```python
from build123d import *

# Parameters (mm, degrees)
F0_R     = 14
F1_DEPTH = 40
F2_R     = 2.5
F3_DEPTH = 15
F4_R     = 2.5
F5_DEPTH = 15


with BuildPart() as f1:
    # F0 (on Front) → F1 (new body)
    with BuildSketch(Plane.XZ):
        Polygon((0, 28), (0, 0), (52, 0), (52, 28), (40, 40), (12, 40), align=None)
        with Locations((26, 20)):
            Circle(F0_R, mode=Mode.SUBTRACT)
    extrude(amount=F1_DEPTH)

    # F2 (on face) → F3 (cut)
    with BuildSketch(Plane.XZ.offset(40)):
        with Locations((39.435029, 33.435029)):
            Circle(F2_R)
        with Locations((45, 20)):
            Circle(F2_R)
        with Locations((39.435029, 6.564971)):
            Circle(F2_R)
        with Locations((12.564971, 6.564971)):
            Circle(F2_R)
        with Locations((7, 20)):
            Circle(F2_R)
        with Locations((12.564971, 33.435029)):
            Circle(F2_R)
    extrude(amount=-F3_DEPTH, mode=Mode.SUBTRACT)

    # F4 (on face) → F5 (cut)
    with BuildSketch(Plane(origin=(0, 0, 0), x_dir=(1, 0, 0), z_dir=(0, 0, -1))):
        with Locations((46, 32)):
            Circle(F4_R)
        with Locations((46, 8)):
            Circle(F4_R)
        with Locations((6, 8)):
            Circle(F4_R)
        with Locations((6, 32)):
            Circle(F4_R)
    extrude(amount=-F5_DEPTH, mode=Mode.SUBTRACT)


solid = f1.part
```
Read the model definition and answer for the solid it produces. Units are mm, in the model's axes. A direction names the side the tool comes from. Coordinates: 2 decimals unless noted, no trailing zeros. Write each loop counter-clockwise with the first axis right and the second up, starting at its lowest first coordinate (ties: lowest second). Pieces come first, ordered by that corner, then holes. Notation, with made-up numbers: (56, 41) - (82, 41) arc R8 ccw to (82, 53) - close; hole circle Ø10 at (81, 48). An arc over 180 degrees is marked (long way). Answer as a JSON object with one key per item and string values. Group by question number.
1. Which of the six approach directions +Z, -Z, +X, -X, +Y, -Y give full straight-line access (tool end or side, diameter ignored) to faces 4 (the cylindrical face through (48.31, -7.04, 7.4)), 5 (the flat face through (6, -20, 34)), 6 (the cylindrical face through (46.34, -32.61, 22.11))?
2. Each of these flat-tipped pins is pushed along its axis until it touches: P1, Ø2.5, axis at x = 13, z = 7.5, coming from the -Y side; P2, Ø2.5, axis at x = 45, y = -32, coming from the -Z side; P3, Ø3, axis at x = 46, y = -32, coming from the +Z side; P4, Ø4, axis at x = 11.5, z = 33, coming from the -Y side. Where does it stop, or does it pass through?
3. A cutting plane is placed at A-A (y = -19). Determine the outline of the cut face in (x, z), plus the area to 3 significant figures.
4. Consider L1, parallel to Y at x = 46, z = 7.75; L2, parallel to X at y = -8, z = 4.5; L3, parallel to Z at x = 26, y = -14. Determine where each line is inside the solid, lowest interval first. Write a range as [from, to].
5. A cutting plane is placed at B-B (x = 23.5). Determine the outline of the cut face in (y, z).
6. A cutting plane is placed at C-C (z = 29). Determine the outline of the cut face in (x, y), plus the area to 3 significant figures.
7. A cutting plane is placed at D-D (y = -33.5). Determine the outline of the cut face in (x, z).
8. The mould has two halves that part along X. Classify faces 1 (the flat face through (46, -20, 34)), 2 (the cylindrical face through (7.34, -34.11, 7.4)), 3 (the flat face through (26, -20, 40)): +X half, -X half, draft (parallel to the pull), parting line (faces both ways), or undercut.
Worked out:
{
 "1": {"face 4": "-Z", "face 5": "+Z, -X, +Y, -Y", "face 6": "-Y"},
 "2": {"P1": "stops at y = -25", "P2": "stops at z = 15", "P3": "stops at z = 35.5", "P4": "stops at y = -40"},
 "3": {"outline": "(0, 0) - (52, 0) - (52, 28) - (40, 40) - (12, 40) - (0, 28) - close; hole circle Ø28 at (26, 20)", "area": "1,320 mm²"},
 "4": {"L1": "y = [-40, -34.5], [-29.5, -10.5], [-5.5, 0]", "L2": "x = [0, 3.5], [8.5, 43.5], [48.5, 52]", "L3": "z = [0, 6], [34, 40]"},
 "5": {"outline": "(-40, 0) - (0, 0) - (0, 6.23) - (-40, 6.23) - close; (-40, 33.77) - (0, 33.77) - (0, 40) - (-40, 40) - close"},
 "6": {"outline": "(1, -40) - (15.28, -40) - (15.28, 0) - (1, 0) - close; (36.72, -40) - (51, -40) - (51, 0) - (36.72, 0) - close", "area": "1,140 mm²"},
 "7": {"outline": "(0, 0) - (4, 0) - (4, 15) - (8, 15) - (8, 0) - (44, 0) - (44, 15) - (48, 15) - (48, 0) - (52, 0) - (52, 28) - (40, 40) - (12, 40) - (0, 28) - close; hole circle Ø5 at (7, 20); hole circle Ø5 at (12.56, 6.56); hole circle Ø5 at (12.56, 33.44); hole circle Ø28 at (26, 20); hole circle Ø5 at (39.44, 6.56); hole circle Ø5 at (39.44, 33.44); hole circle Ø5 at (45, 20)"},
 "8": {"face 1": "+X half", "face 2": "undercut", "face 3": "draft"}
}
